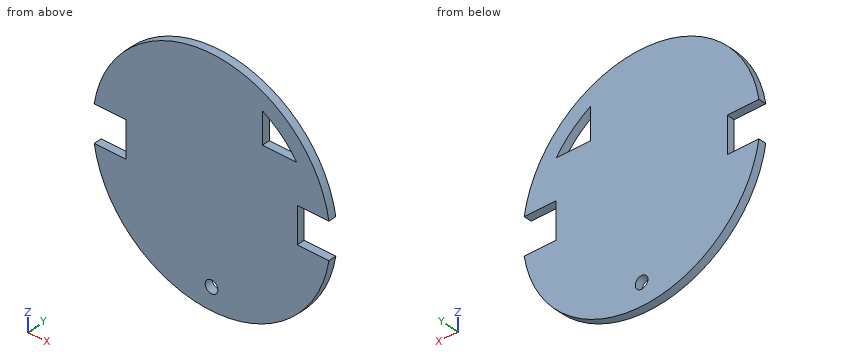
from build123d import *

# Parameters (mm, degrees)
SKETCH1_R           = 75
BOSS_EXTRUDE1_DEPTH = 5
SKETCH2_R           = 4
CUT_EXTRUDE1_DEPTH  = 5


with BuildPart() as part:
    # Sketch1 → Boss-Extrude1 (new body)
    with BuildSketch(Plane(origin=(0, 0, 0), x_dir=(1, 0, 0), z_dir=(0, 1, 0))):
        with Locations((-5.935816789, 0)):
            Circle(SKETCH1_R)
    extrude(amount=BOSS_EXTRUDE1_DEPTH)

    # Sketch2 → Cut-Extrude1 (cut)
    with BuildSketch(Plane(origin=(0, 5, 0), x_dir=(1, 0, 0), z_dir=(0, 1, 0))):
        with BuildLine():
            ThreePointArc((-80.048906052, -11.5), (-80.935816789, 0), (-80.048906052, 11.5))
            Line((-80.048906052, 11.5), (-89.004044114, 11.5))
            Line((-89.004044114, 11.5), (-89.004044114, -11.5))
            Line((-89.004044114, -11.5), (-80.048906052, -11.5))
        make_face()
        with BuildLine():
            Line((-69.910421126, 11.5), (-80.048906052, 11.5))
            Line((-80.048906052, 11.5), (-80.048906052, -11.5))
            Line((-80.048906052, -11.5), (-69.910421126, -11.5))
            ThreePointArc((-69.910421126, -11.5), (-70.935816789, 0), (-69.910421126, 11.5))
        make_face()
        with BuildLine():
            Line((-60.048906052, 11.5), (-69.910421126, 11.5))
            ThreePointArc((-69.910421126, 11.5), (-70.935816789, 0), (-69.910421126, -11.5))
            Line((-69.910421126, -11.5), (-60.048906052, -11.5))
            Line((-60.048906052, -11.5), (-60.048906052, 11.5))
        make_face()
        with BuildLine():
            ThreePointArc((59.064183211, 0), (58.807326793, 5.772812059), (58.038787547, 11.5))
            Line((58.038787547, 11.5), (48.177272473, 11.5))
            Line((48.177272473, 11.5), (48.177272473, -11.5))
            Line((48.177272473, -11.5), (58.038787547, -11.5))
            ThreePointArc((58.038787547, -11.5), (58.807326793, -5.772812059), (59.064183211, 0))
        make_face()
        with BuildLine():
            Line((68.177272473, -11.5), (68.177272473, 11.5))
            Line((68.177272473, 11.5), (58.038787547, 11.5))
            ThreePointArc((58.038787547, 11.5), (58.807326793, 5.772812059), (59.064183211, 0))
            ThreePointArc((59.064183211, 0), (58.807326793, -5.772812059), (58.038787547, -11.5))
            Line((58.038787547, -11.5), (68.177272473, -11.5))
        make_face()
        with BuildLine():
            Line((83.116270972, 11.5), (68.177272473, 11.5))
            ThreePointArc((68.177272473, 11.5), (68.842126799, 5.767074879), (69.064183211, 0))
            ThreePointArc((69.064183211, 0), (68.842126799, -5.767074879), (68.177272473, -11.5))
            Line((68.177272473, -11.5), (83.116270972, -11.5))
            Line((83.116270972, -11.5), (83.116270972, 11.5))
        make_face()
        with BuildLine():
            Line((26.200611139, -36.5), (26.200611139, -56.5))
            ThreePointArc((26.200611139, -56.5), (38.173054222, -47.743140849), (47.848474598, -36.5))
            Line((47.848474598, -36.5), (26.200611139, -36.5))
        make_face()
        with Locations((-5.948906052, 60.999998596)):
            Circle(SKETCH2_R)
        with BuildLine():
            Line((-80.048906052, -11.5), (-80.048906052, 11.5))
            ThreePointArc((-80.048906052, 11.5), (-80.935816789, 0), (-80.048906052, -11.5))
        make_face()
        with BuildLine():
            ThreePointArc((69.064183211, 0), (68.842126799, 5.767074879), (68.177272473, 11.5))
            Line((68.177272473, 11.5), (68.177272473, -11.5))
            ThreePointArc((68.177272473, -11.5), (68.842126799, -5.767074879), (69.064183211, 0))
        make_face()
    extrude(amount=-CUT_EXTRUDE1_DEPTH, mode=Mode.SUBTRACT)


solid = part.part
Input: part model. Units: mm. Frame: model coordinates. Coordinates: 2 decimals unless noted, no trailing zeros. Loops run counter-clockwise (first coordinate to the right, second up) from the corner with the lowest first, then second, coordinate; pieces in that order, holes last. Notation, with made-up numbers: (-4, 38.5) - (35, 38.5) arc R7 ccw to (35, 45.5) - close; hole circle Ø5 at (-40, -15.75). An arc over 180 degrees is marked (long way). Answer in a Markdown table with one row per item. Add a question column.
Item 1: Section query A-A on y = 3.2. Return the cut outline in (x, z), then the cut area to 3 significant figures.
Item 2: Section query C-C on z = -8.5. Return the cut outline in (x, y), then the cut area to 3 significant figures.
Item 3: Section query B-B on x = 55. Return the cut outline in (y, z), then the cut area to 3 significant figures.
Item 4: Contact query for flat-ended pins moving along their axis: P1, Ø2.5, axis at y = 2, z = -4.5, coming from the -X side; P2, Ø2.5, axis at x = -73, y = 3, coming from the -Z side; P3, Ø12, axis at x = -62, z = -57, coming from the -Y side; P4, Ø2.5, axis at x = -65.5, y = 3.5, coming from the +Z side. Output: stop coordinate, or through.
Item 5: Line query: line 1 along Z through (x, y) = (-7.5, 0.55); line 2 along Z through (x, y) = (28, 4.2); line 3 along X through (y, z) = (2.55, -3). Output: solid intervals per line, ascending. Write a range as [from, to].
Item 6: Section query D-D on x = 32. Return the cut outline in (y, z).
Recorded:
| question | item | result |
|---|---|---|
| 1 | outline | (-80.05, -11.5) arc R75 ccw to (68.18, -11.5) - (48.18, -11.5) - (48.18, 11.5) - (68.18, 11.5) arc R75 ccw to (-80.05, 11.5) - (-60.05, 11.5) - (-60.05, -11.5) - close; hole circle Ø8 at (-5.95, -61); hole (26.2, 36.5) - (47.85, 36.5) arc R65 ccw to (26.2, 56.5) - close |
| 1 | area | 16,400 mm^2 |
| 2 | outline | (-60.05, 0) - (48.18, 0) - (48.18, 5) - (-60.05, 5) - close |
| 2 | area | 541 mm^2 |
| 3 | outline | (0, -43.72) - (5, -43.72) - (5, -11.5) - (0, -11.5) - close; (0, 11.5) - (5, 11.5) - (5, 43.72) - (0, 43.72) - close |
| 3 | area | 322 mm^2 |
| 4 | P1 | x = -60.05 |
| 4 | P2 | z = -35.97 |
| 4 | P3 | y = 0 |
| 4 | P4 | z = 47.16 |
| 5 | line 1 | [-74.98, -64.69], [-57.31, 74.98] |
| 5 | line 2 | [-66.88, 36.5], [55.44, 66.88] |
| 5 | line 3 | [-60.05, 48.18] |
| 6 | outline | (0, -64.7) - (5, -64.7) - (5, 36.5) - (0, 36.5) - close; (0, 52.78) - (5, 52.78) - (5, 64.7) - (0, 64.7) - close |
